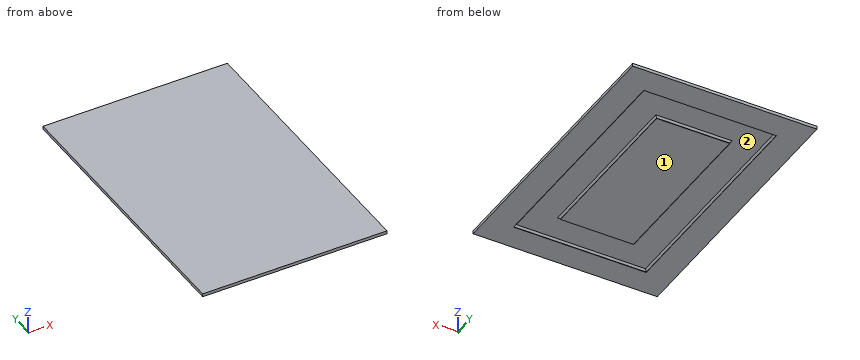
```python
from build123d import *

# Parameters (mm, degrees)
SKETCH1_W          = 415
SKETCH1_H          = 630
BASE_EXTRUDE_DEPTH = 7
SKETCH19_W         = 298.8
SKETCH19_H         = 513.8
SKETCH19_W_2       = 164.4
SKETCH19_H_2       = 379.4
CUT_EXTRUDE1_DEPTH = 5
CHAMFER1_SIZE      = 4


with BuildPart() as part:
    # Sketch1 → Base-Extrude (new body)
    with BuildSketch(Plane.XY):
        with Locations((207.5, 315)):
            Rectangle(SKETCH1_W, SKETCH1_H)
    extrude(amount=BASE_EXTRUDE_DEPTH)

    # Sketch19 → Cut-Extrude1 (cut)
    with BuildSketch(Plane(origin=(0, 0, 0), x_dir=(-1, 0, 0), z_dir=(0, 0, -1))):
        with Locations((-207.5, 315)):
            Rectangle(SKETCH19_W, SKETCH19_H)
        with Locations((-207.5, 315)):
            Rectangle(SKETCH19_W_2, SKETCH19_H_2, mode=Mode.SUBTRACT)
    extrude(amount=-CUT_EXTRUDE1_DEPTH, mode=Mode.SUBTRACT)

    # Chamfer1
    chamfer1_edges = [part.edges().sort_by_distance(p)[0] for p in [
        (207.5, 58.1, 5),
        (356.9, 315, 5),
        (207.5, 571.9, 5),
        (58.1, 315, 5),
        (289.7, 315, 5),
        (207.5, 125.3, 5),
        (125.3, 315, 5),
        (207.5, 504.7, 5),
    ]]
    chamfer(chamfer1_edges, length=CHAMFER1_SIZE)


solid = part.part
```
Geometry: final body of the model. Coordinates: model frame, mm. Face numbers are marked on the shaded views. Round coordinates to 2 decimals unless told otherwise and drop trailing zeros. Write each loop counter-clockwise with the first axis right and the second up, starting at its lowest first coordinate (ties: lowest second). Pieces come first, ordered by that corner, then holes.
Item 1: Section query B-B (y = 558). Return loops of the section in (x, z).
Item 2: Section query A-A (z = 2.5). Return loops of the section in (x, y), plus the area to 3 significant figures.
Item 3: Section query D-D (y = 177.5). Return loops of the section in (x, z), plus the area to 4 significant figures.
Item 4: Mould query, pull axis X, two halves, no side actions, for the marked faces 1 and 2. Classes: +X half, -X half, draft (parallel to the pull), parting line (faces both ways), or undercut.
Item 5: Material intervals for L1, parallel to X at y = 534, z = 0.5; L2, parallel to Y at x = 217.5, z = 2.5; L3, parallel to Y at x = 288, z = 1.75, sorted ascending.
Item 6: Section query C-C (x = 205). Return loops of the section in (y, z).
Completed:
1. outline: (0, 0) - (58.1, 0) - (58.1, 1) - (62.1, 5) - (352.9, 5) - (356.9, 1) - (356.9, 0) - (415, 0) - (415, 7) - (0, 7) - close
2. outline: (0, 0) - (415, 0) - (415, 630) - (0, 630) - close; (123.8, 123.8) - (291.2, 123.8) - (291.2, 506.2) - (123.8, 506.2) - close; hole (59.6, 59.6) - (355.4, 59.6) - (355.4, 570.4) - (59.6, 570.4) - close
2. area: 174,000 mm2
3. outline: (0, 0) - (58.1, 0) - (58.1, 1) - (62.1, 5) - (121.3, 5) - (125.3, 1) - (125.3, 0) - (289.7, 0) - (289.7, 1) - (293.7, 5) - (352.9, 5) - (356.9, 1) - (356.9, 0) - (415, 0) - (415, 7) - (0, 7) - close
3. area: 2,265 mm2
4. face 1: draft
4. face 2: undercut
5. L1: x = 0 to 58.1, 356.9 to 415
5. L2: y = 0 to 59.6, 123.8 to 506.2, 570.4 to 630
5. L3: y = 0 to 58.85, 124.55 to 505.45, 571.15 to 630
6. outline: (0, 0) - (58.1, 0) - (58.1, 1) - (62.1, 5) - (121.3, 5) - (125.3, 1) - (125.3, 0) - (504.7, 0) - (504.7, 1) - (508.7, 5) - (567.9, 5) - (571.9, 1) - (571.9, 0) - (630, 0) - (630, 7) - (0, 7) - close
